Autodesk Inventor part; units mm, degrees
ref_plane "YZ Plane" through (0, 0, 0) normal (1, 0, 0) x (0, 1, 0)
ref_plane "XZ Plane" through (0, 0, 0) normal (0, 1, 0) x (-1, 0, 0)
ref_plane "XY Plane" through (0, 0, 0) normal (0, 0, 1) x (1, 0, 0)
sketch "スケッチ1" plane through (0, 0, 0) normal (0, 1, 0) x (-1, 0, 0)
  arc A0 (-44.6969, -164.0189) -> (44.6969, -164.0189) centre (0, 0) ccw
  arc A1 (-43.0967, -158.2361) -> (43.0967, -158.2361) centre (0, 0) ccw
  line L0 (45.5455, -159.6171) -> (46.0943, -161.5404)
  line L1 (-45.5455, -159.6171) -> (-46.0943, -161.5404)
  arc A2 (44.6969, -164.0189) -> (46.0943, -161.5404) centre (44.1711, -162.0892) ccw
  arc A3 (45.5455, -159.6171) -> (43.0967, -158.2361) centre (43.6222, -160.1659) ccw
  arc A4 (-43.0967, -158.2361) -> (-45.5455, -159.6171) centre (-43.6222, -160.1659) ccw
  arc A5 (-46.0943, -161.5404) -> (-44.6969, -164.0189) centre (-44.1711, -162.0892) ccw
  line L2 (0, -204) -> (0, 34)
  point P0 (-46.6463, -163.4751)
  point P1 (46.6463, -163.4751)
  point P2 (-45, -157.7054)
  point P3 (45, -157.7054)
  point P4 (-46.6463, -163.4751)
  dimension "d0" = 170
  dimension "d1" = 6
  dimension "d2" = 2
  dimension "d3" = 90
extrude "押し出し1" add sketch "スケッチ1" along normal blind 2
properties part number "SubHandle"
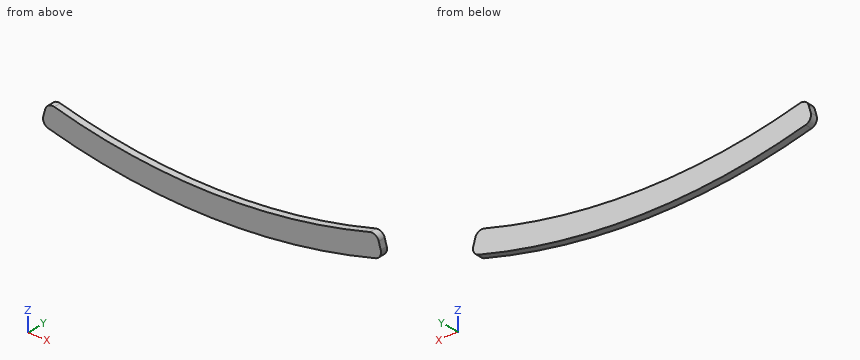
Geometry: final body of the model. Coordinates: model frame, mm. Round coordinates to 2 decimals unless told otherwise and drop trailing zeros. Loops run counter-clockwise (first coordinate to the right, second up) from the corner with the lowest first, then second, coordinate; pieces in that order, holes last. Notation, with made-up numbers: (1, 81) -> (14, 81) arc R21 cw to (14, 102) -> close; hole circle Ø8 at (18, 26). An arc over 180 degrees is marked (long way). Use one line per item in the form item = value. Start each with the question number.
1) Section A-A on y = 0.4. Output: boundary loops of the cut face in (x, z), then the cut area to 3 significant figures.
2) First-contact query: P1, Ø5, axis at x = 0.5, z = -160.5, coming from the +Y side. Flat tip, straight axial feed; report the tip coordinate or a pass-through.
3) Line query: L1, parallel to Z at x = 6, y = 0.75; L2, parallel to Z at x = 41, y = 0.2. Output: solid intervals per line, ascending.
4) Section C-C on x = 39. Output: boundary loops of the cut face in (y, z).
5) Section B-B on z = -162.75. Output: boundary loops of the cut face in (x, y), then the cut area to 3 significant figures.
6) Section D-D on z = -166.5. Output: boundary loops of the cut face in (x, y).
Response:
q1.outline = (-46.09, -161.54) arc R2 ccw to (-44.7, -164.02) arc R170 ccw to (44.7, -164.02) arc R2 ccw to (46.09, -161.54) -> (45.55, -159.62) arc R2 ccw to (43.1, -158.24) arc R164 cw to (-43.1, -158.24) arc R2 ccw to (-45.55, -159.62) -> close
q1.area = 554 mm^2
q2.P1 = through
q3.L1 = -169.89 to -163.89
q3.L2 = -164.98 to -158.79
q4.outline = (0, -165.47) -> (2, -165.47) -> (2, -159.3) -> (0, -159.3) -> close
q5.outline = (-46.06, 0) -> (-20.21, 0) -> (-20.21, 2) -> (-46.06, 2) -> close; (20.21, 0) -> (46.06, 0) -> (46.06, 2) -> (20.21, 2) -> close
q5.area = 103 mm^2
q6.outline = (-34.32, 0) -> (34.32, 0) -> (34.32, 2) -> (-34.32, 2) -> close
